Geometry: final body of the model. Coordinates: model frame, mm. A direction names the side the tool comes from. Give positions to 0.01 mm unless a question says otherwise; leave off trailing zeros. Write each loop counter-clockwise with the first axis right and the second up, starting at its lowest first coordinate (ties: lowest second). Pieces come first, ordered by that corner, then holes. Notation, with made-up numbers: (39, 88) -> (65, 88) arc R24 ccw to (65, 106) -> close; hole circle Ø7 at (-2, 54). An arc over 180 degrees is marked (long way). Answer as a JSON object with one key per item and string values.
from build123d import *

# Parameters (mm, degrees)
SKETCH1_R           = 15
SKETCH1_R_2         = 6
BOSS_EXTRUDE1_DEPTH = 25


with BuildPart() as part:
    # Sketch1 → Boss-Extrude1 (new body)
    with BuildSketch(Plane.XY):
        with BuildLine():
            Line((40.063427207, -29.949425047), (64.999534256, -29.955194996))
            ThreePointArc((64.999534256, -29.955194996), (72.069106212, -32.884945049), (74.997220362, -39.955194729))
            Line((74.997220362, -39.955194729), (74.997220362, -59.917750729))
            Line((74.997220362, -59.917750729), (-80.002779638, -59.917750729))
            Line((-80.002779638, -59.917750729), (-80.002779638, 50.082249271))
            ThreePointArc((-80.002779638, 50.082249271), (-77.073847449, 57.153317083), (-70.002779638, 60.082249271))
            Line((-70.002779638, 60.082249271), (-30.002779638, 60.082249271))
            ThreePointArc((-30.002779638, 60.082249271), (-22.931711826, 57.153317083), (-20.002779638, 50.082249271))
            Line((-20.002779638, 50.082249271), (-20.002779638, 39.24305603))
            ThreePointArc((-20.002779638, 39.24305603), (-17.640405796, 32.788083786), (-11.669446304, 29.382923058))
            ThreePointArc((-11.669446304, 29.382923058), (18.22116437, 12.344839461), (30.065744482, -19.957649933))
            ThreePointArc((30.065744482, -19.957649933), (32.996763354, -27.022582575), (40.063427207, -29.949425047))
        make_face()
        with Locations((-50, 40.082249271)):
            Circle(SKETCH1_R, mode=Mode.SUBTRACT)
        with Locations((-60.002779638, -44.917750729)):
            Circle(SKETCH1_R_2, mode=Mode.SUBTRACT)
        with Locations((-40.002779638, -44.917750729)):
            Circle(SKETCH1_R_2, mode=Mode.SUBTRACT)
        with Locations((-20.002779638, -44.917750729)):
            Circle(SKETCH1_R_2, mode=Mode.SUBTRACT)
        with Locations((-0.002779638, -44.917750729)):
            Circle(SKETCH1_R_2, mode=Mode.SUBTRACT)
        with Locations((19.997220362, -44.917750729)):
            Circle(SKETCH1_R_2, mode=Mode.SUBTRACT)
        with Locations((39.997220362, -44.917750729)):
            Circle(SKETCH1_R_2, mode=Mode.SUBTRACT)
        with Locations((59.997220362, -44.917750729)):
            Circle(SKETCH1_R_2, mode=Mode.SUBTRACT)
        with BuildLine():
            Line((-15.002779638, 9.662657115), (-50.002779638, 9.662657115))
            ThreePointArc((-50.002779638, 9.662657115), (-57.073847449, 6.733724927), (-60.002779638, -0.337342885))
            Line((-60.002779638, -0.337342885), (-60.002779638, -9.996302817))
            ThreePointArc((-60.002779638, -9.996302817), (-57.072540419, -17.068677418), (-49.999083138, -19.996302134))
            Line((-49.999083138, -19.996302134), (-2.608906127, -19.978784358))
            ThreePointArc((-2.608906127, -19.978784358), (6.045547234, -14.982427813), (6.053700131, -4.989276396))
            ThreePointArc((6.053700131, -4.989276396), (-2.834464117, 4.693663889), (-15.002779638, 9.662657115))
        make_face(mode=Mode.SUBTRACT)
    extrude(amount=BOSS_EXTRUDE1_DEPTH)


solid = part.part
Q1. Material intervals for L1, parallel to Y at x = -50.5, z = 16.5; L2, parallel to Y at x = -49, z = 15.5; L3, parallel to Y at x = -58, z = 21.5, sorted ascending. Write a range as from..to.
Values:
{"L1": "-59.92..-19.98, 9.65..25.09, 55.07..60.08", "L2": "-59.92..-20, 9.66..25.12, 55.05..60.08", "L3": "-59.92..-50.57, -39.26..-16, 5.67..27.39, 52.77..60.08"}
Q2. Cut plane A-A (y = 5). Return the cut outline in (x, z).
Values:
{"outline": "(-80, 0) -> (-58.46, 0) -> (-58.46, 25) -> (-80, 25) -> close; (-3.28, 0) -> (23.38, 0) -> (23.38, 25) -> (-3.28, 25) -> close"}
Q3. Cut plane B-B (z = 4.5). State how many separate pieces and enclosed holes the cut face has, and give its area (3 significant figures).
Values:
{"separate pieces": "1", "enclosed holes": "9", "area": "9,180 mm²"}
Q4. Set-up query: faces 5 (the cylindrical face through (-56.996, 6.811, 12.325)), 6 (the flat face through (-20.003, 45, 12)), 7 (the flat face through (-19, -26, 0)). Return all of +Z, -Z, +X, -X, +Y, -Y with unobstructed straight access to the full face (end or side cutting, diameter ignored); none if empty.
Values:
{"face 5": "+Z, -Z", "face 6": "+Z, -Z, +X, +Y", "face 7": "-Z, +X, -X, +Y, -Y"}
Q5. Mould query, pull axis Y, two halves, no side actions, for faces 1 (the cylindrical face through (5.97, -15.11, 12.32)), 2 (the cylindrical face through (-16.777, -39.859, 12.325)), 3 (the cylindrical face through (-23.01, 57.23, 12.32)), 4 (the flat face through (-1, -59.918, 12)). Classes: pulls with the +Y half, pulls with the -Y half, needs draft (parallel to the pull), parting line crosses it, or undercut.
Values:
{"face 1": "undercut", "face 2": "undercut", "face 3": "pulls with the +Y half", "face 4": "pulls with the -Y half"}
Q6. Cut plane C-C (x = 17). Return the cut outline in (y, z).
Values:
{"outline": "(-59.92, 0) -> (-50.12, 0) -> (-50.12, 25) -> (-59.92, 25) -> close; (-39.72, 0) -> (13.74, 0) -> (13.74, 25) -> (-39.72, 25) -> close"}
Q7. First-contact query: P1, Ø12, axis at y = 44, z = 9.5, coming from the +X side; P2, Ø10.5, axis at y = -7.5, z = 15.5, coming from the +X side. Flat tips, straight axial feed; report the tip coordinate or a pass-through.
Values:
{"P1": "x = -19.93", "P2": "x = 29.54"}
Q8. Cut plane D-D (y = -23.5). Return the cut outline in (x, z).
Values:
{"outline": "(-80, 0) -> (30.72, 0) -> (30.72, 25) -> (-80, 25) -> close"}
